Model file for the job. Use its own axes, mm. A direction names the side the tool comes from. Round coordinates to 2 decimals unless told otherwise and drop trailing zeros. Loops run counter-clockwise (first coordinate to the right, second up) from the corner with the lowest first, then second, coordinate; pieces in that order, holes last. Notation, with made-up numbers: (33, -40) -> (57, -40) arc R19 cw to (57, -19) -> close; hole circle Ø6 at (67.25, 1). An arc over 180 degrees is marked (long way). Use a Markdown table: item, result.
from build123d import *

# Parameters (mm, degrees)
F1_DEPTH = 3
F2_DEPTH = 15
F3_DEPTH = 9


with BuildPart() as f1:
    # F0 (on Top) → F1 (new body)
    with BuildSketch(Plane.XY):
        with BuildLine():
            ThreePointArc((-4.4288796676, -3.6796678124), (-2.3253257096, -2.3633430927), (-1.5043057066, -0.0216394017))
            ThreePointArc((-1.5043057066, -0.0216394017), (-2.3253257096, 2.3200642894), (-4.4288796676, 3.6363890091))
            ThreePointArc((-4.4288796676, 3.6363890091), (-9.0043057066, -0.0216394017), (-4.4288796676, -3.6796678124))
        make_face()
        with BuildLine():
            ThreePointArc((-4.4288796676, 3.6363890091), (-2.3253257096, 2.3200642894), (-1.5043057066, -0.0216394017))
            ThreePointArc((-1.5043057066, -0.0216394017), (-2.3253257096, -2.3633430927), (-4.4288796676, -3.6796678124))
            Line((-4.4288796676, -3.6796678124), (5.7708010962, -2.262551744))
            ThreePointArc((5.7708010962, -2.262551744), (3.4956906544, -0.0126918671), (5.7708010962, 2.2371680098))
            Line((5.7708010962, 2.2371680098), (-4.4288796676, 3.6363890091))
        make_face()
        with BuildLine():
            ThreePointArc((7.9956906544, -0.0126918671), (7.3455341614, 1.5693955998), (5.7708010962, 2.2371680098))
            ThreePointArc((5.7708010962, 2.2371680098), (3.4956906544, -0.0126918671), (5.7708010962, -2.262551744))
            ThreePointArc((5.7708010962, -2.262551744), (7.3455341614, -1.594779334), (7.9956906544, -0.0126918671))
        make_face()
    extrude(amount=F1_DEPTH)

    # F0 (on Top) → F2 (join)
    with BuildSketch(Plane.XY):
        with BuildLine():
            ThreePointArc((-4.4288796676, -3.6796678124), (-2.3253257096, -2.3633430927), (-1.5043057066, -0.0216394017))
            ThreePointArc((-1.5043057066, -0.0216394017), (-2.3253257096, 2.3200642894), (-4.4288796676, 3.6363890091))
            ThreePointArc((-4.4288796676, 3.6363890091), (-9.0043057066, -0.0216394017), (-4.4288796676, -3.6796678124))
        make_face()
    extrude(amount=F2_DEPTH)

    # F0 (on Top) → F3 (join)
    with BuildSketch(Plane.XY):
        with BuildLine():
            ThreePointArc((7.9956906544, -0.0126918671), (7.3455341614, 1.5693955998), (5.7708010962, 2.2371680098))
            ThreePointArc((5.7708010962, 2.2371680098), (3.4956906544, -0.0126918671), (5.7708010962, -2.262551744))
            ThreePointArc((5.7708010962, -2.262551744), (7.3455341614, -1.594779334), (7.9956906544, -0.0126918671))
        make_face()
    extrude(amount=F3_DEPTH)


solid = f1.part
Q1. Pull direction X, two halves, no side cores. Call faces 4 (the face through (7.973, 0.305, 5.437)), 5 (the face through (-1, 0, 0)), 6 (the face through (1, 0, 3)), 7 (the face through (0.742, 2.927, 1.479)): released by +X, released by -X, zero draft, split by the parting line, or undercut.
Results list:
| item | result |
|---|---|
| face 4 | undercut |
| face 5 | zero draft |
| face 6 | undercut |
| face 7 | released by +X |
Q2. Tool access for faces 1 (the face through (6, 0, 9)), 2 (the face through (0.6, -2.98, 1.48)), 3 (the face through (-9.004, -0.034, 7.395)): list every direction of +Z, -Z, +X, -X, +Y, -Y with a clear straight run to the whole face (end or side of a thin tool).
Results list:
| item | result |
|---|---|
| face 1 | +Z, +X, +Y, -Y |
| face 2 | +Z, -Z, +X, -Y |
| face 3 | +Z |
Q3. Band-saw the part on B-B, the plane x = 4.25. Give the cut face in (y, z), plus the area to 3 significant figures.
Results list:
| item | result |
|---|---|
| outline | (-2.47, 0) -> (2.45, 0) -> (2.45, 3) -> (1.67, 3) -> (1.67, 9) -> (-1.69, 9) -> (-1.69, 3) -> (-2.47, 3) -> close |
| area | 34.9 mm² |
Q4. Flat gauge pins, fed straight in: pin 1 (1.5 mm diameter, centred on x = -4, z = 11, fed in from -Y); pin 2 (3.5 mm diameter, centred on x = 6, y = -0.5, fed in from +Z); pin 3 (2 mm diameter, centred on x = 0, y = 1, fed in from +Z). Where does each tip first touch, or does it go through?
Results list:
| item | result |
|---|---|
| pin 1 | stops at y = -3.74 |
| pin 2 | stops at z = 9 |
| pin 3 | stops at z = 3 |
Q5. Drill centre lines: L1, parallel to Z at x = 0, y = 2.5; L2, parallel to X at y = 0, z = 3.75; L3, parallel to X at y = 0, z = 13. Where is each one in solid material? Low to high. Write a range as from..to.
Results list:
| item | result |
|---|---|
| L1 | z = 0..3 |
| L2 | x = -9..-1.5, 3.5..8 |
| L3 | x = -9..-1.5 |
Q6. Band-saw the part on A-A, the plane z = 5.75. Give the cut face in (x, y).
Results list:
| item | result |
|---|---|
| outline | circle Ø7.5 at (-5.25, -0.02); circle Ø4.5 at (5.75, -0.01) |
Q7. Band-saw the part on D-D, the plane z = 2.5. Give the cut face in (x, y), plus the area to 3 significant figures.
Results list:
| item | result |
|---|---|
| outline | (-4.43, -3.68) -> (5.77, -2.26) arc R2.25 ccw to (5.77, 2.24) -> (-4.43, 3.64) arc R3.75 ccw (long way) to start |
| area | 96.3 mm² |
Q8. Band-saw the part on C-C, the plane y = 1.5. Give the cut face in (x, z).
Results list:
| item | result |
|---|---|
| outline | (-8.68, 0) -> (7.41, 0) -> (7.41, 9) -> (4.08, 9) -> (4.08, 3) -> (-1.83, 3) -> (-1.83, 15) -> (-8.68, 15) -> close |
